```python
from build123d import *

# Parameters (mm, degrees)
F0_W          = 82.8472673893
F0_H          = 84.5430567861
F1_DEPTH      = 25
F3_DEPTH      = 215.0975316763
F3_TAPER      = -3
F3_DEPTH_BACK = 25


with BuildPart() as f1:
    # F0 (on Top) → F1 (new body)
    with BuildSketch(Plane.XY):
        with Locations((41.4236336946, 42.271528393)):
            Rectangle(F0_W, F0_H)
    extrude(amount=F1_DEPTH)

    # F2 (on face) → F3 (cut, two sides)
    with BuildSketch(Plane.XY.offset(25)) as f3_sk:
        Polygon((66.8386592076, 29.4964735825), (64.8125708103, 59.0836033225), (38.1763206318, 72.1225241702), (13.5661588504, 55.5743152778), (15.5922472477, 25.9871855378), (42.2284974263, 12.9482646901), align=None)
    extrude(amount=F3_DEPTH, taper=F3_TAPER, mode=Mode.SUBTRACT)
    extrude(f3_sk.sketch, amount=-F3_DEPTH_BACK, mode=Mode.SUBTRACT)


solid = f1.part
```
Verification items for the finished model (mm, model axes). A direction names the side the tool comes from. Give positions to 0.01 mm unless a question says otherwise; leave off trailing zeros. Loops run counter-clockwise (first coordinate to the right, second up) from the corner with the lowest first, then second, coordinate; pieces in that order, holes last. Notation, with made-up numbers: M 81,-1 L 94,-1 A22 cw 94,16 Z; hole C 75,-5 d11. An arc over 180 degrees is marked long. Return JSON: item names as keys, results as strings.
1) Section check C-C, the plane y = 21.5. Enter the section's corners in (x, z), and give its area (3 significant figures).
Findings:
{"outline": "M 0,0 L 24.76,0 L 24.76,25 L 0,25 Z; M 54.95,0 L 82.85,0 L 82.85,25 L 54.95,25 Z", "area": "1,320 mm2"}
2) Section check B-B, the plane x = 23. Enter the section's corners in (y, z).
Findings:
{"outline": "M 0,0 L 22.36,0 L 22.36,25 L 0,25 Z; M 61.92,0 L 84.54,0 L 84.54,25 L 61.92,25 Z"}
3) Section check A-A, the plane z = 15. Enter the section's corners in (x, y), and give its area (3 significant figures).
Findings:
{"outline": "M 0,0 L 82.85,0 L 82.85,84.54 L 0,84.54 Z; hole M 13.57,55.57 L 15.59,25.99 L 42.23,12.95 L 66.84,29.5 L 64.81,59.08 L 38.18,72.12 Z", "area": "4,720 mm2"}
4) Tool access check on faces 1 (the flat face through (14.565, 40.988, 12.675)), 2 (the flat face through (0, 42, 12)). Record the directions out of +Z, -Z, +X, -X, +Y, -Y that give a thin tool (end or side, any length) a straight path to the whole face; none if there is none.
Findings:
{"face 1": "+Z, -Z", "face 2": "+Z, -Z, -X, +Y, -Y"}
5) Material ranges on L1, parallel to X at y = 57, z = 13.5; L2, parallel to Y at x = 18, z = 16; L3, parallel to Y at x = 44.5, z = 19.5, recorded low to high. Write a range as [from, to].
Findings:
{"L1": "x = [0, 15.69], [64.96, 82.85]", "L2": "y = [0, 24.81], [58.56, 84.54]", "L3": "y = [0, 14.48], [69.03, 84.54]"}
